Autodesk Inventor part; units mm, degrees
ref_plane "YZ Plane" through (0, 0, 0) normal (1, 0, 0) x (0, 1, 0)
ref_plane "XZ Plane" through (0, 0, 0) normal (0, 1, 0) x (-1, 0, 0)
ref_plane "XY Plane" through (0, 0, 0) normal (0, 0, 1) x (1, 0, 0)
sketch "Sketch1" plane through (0, 0, 0) normal (0, 0, 1) x (1, 0, 0)
  circle A0 centre (-23.5281, 14.2673) radius 2.25
  circle A1 centre (-21.1834, 86.2291) radius 2.25
  arc A2 (-21.1834, 86.2291) -> (-23.5281, 14.2673) centre (131.108, 45.2479) ccw construction
  arc A3 (-25.046, 87.2685) -> (-27.4502, 13.4815) centre (131.108, 45.2479) ccw
  arc A4 (-17.3208, 85.1897) -> (-19.6061, 15.053) centre (131.108, 45.2479) ccw
  arc A5 (-17.3208, 85.1897) -> (-25.046, 87.2685) centre (-21.1834, 86.2291) ccw
  arc A6 (-27.4502, 13.4815) -> (-19.6061, 15.053) centre (-23.5281, 14.2673) ccw
  point P0 (0, 0)
  dimension "d0" = 8
extrude "Extrusion1" add sketch "Sketch1" along normal blind 9
scale "Scale1" factors (0.5, 0.5, 0.5) then translate (65.554, 22.624, 2.25) bodies 1
properties part number "MasiveBone2"
Read the model definition and answer for the solid it produces. Units are mm, in the model's axes. Round coordinates to 2 decimals unless told otherwise and drop trailing zeros. Write each loop counter-clockwise with the first axis right and the second up, starting at its lowest first coordinate (ties: lowest second). Pieces come first, ordered by that corner, then holes.
1. Determine the mould class of faces 1 (the face through (54.2, 27.8, 4.5)), 2 (the face through (55.481, 66.737, 4.469)), 3 (the face through (53, 48, 2.25)), 4 (the face through (52.666, 29.708, 4.469)) for opening direction X: pulls with the +X half, pulls with the -X half, needs draft (parallel to the pull), parting line crosses it, or undercut.
2. The part is cut by section C-C, the plane y = 55.5. Determine the outline of the cut face in (x, z), then the cut area to 3 significant figures.
3. The part is cut by section B-B, the plane y = 45. Determine the outline of the cut face in (x, z).
4. The part is cut by section A-A, the plane z = 3.85. State how many separate pieces and enclosed holes the cut face has, then the cut area to 3 significant figures.
5. Given pin 1 Ø1 at (y, z) = (39.5, 4.5) entering from +X; pin 2 Ø1.8 at (x, y) = (53.79, 29.76) entering from +Z; pin 3 Ø2 at (y, z) = (35, 5.5) entering from +X; pin 4 Ø2 at (y, z) = (53.5, 6) entering from -X, each flat-ended and moving along its own axis, determine where each tip first touches the part or whether it passes through.
6. Straight lines are drawn through the part: L1, parallel to Y at x = 53.5, z = 3.55; L2, parallel to X at y = 65.5, z = 2.5; L3, parallel to X at y = 66, z = 4.9. For each, find the intervals that lie inside material, in ascending order.
Values:
1. face 1: parting line crosses it
1. face 2: undercut
1. face 3: needs draft
1. face 4: undercut
2. outline: (50.91, 2.25) - (54.94, 2.25) - (54.94, 6.75) - (50.91, 6.75) - close
2. area: 18.2 mm2
3. outline: (50.25, 2.25) - (54.25, 2.25) - (54.25, 6.75) - (50.25, 6.75) - close
4. separate pieces: 1
4. enclosed holes: 2
4. area: 150 mm2
5. pin 1: stops at x = 54.51
5. pin 2: passes through
5. pin 3: stops at x = 55.08
5. pin 4: stops at x = 50.58
6. L1: y = 27.78 to 28.67, 30.84 to 67.1
6. L2: x = 52.83 to 53.86, 56.06 to 56.95
6. L3: x = 52.96 to 53.87, 56.06 to 56.95
